The listing builds one solid part. Answer for the finished solid, in the listing's coordinates (mm). A direction names the side the tool comes from. Coordinates: 2 decimals unless noted, no trailing zeros. Loops run counter-clockwise (first coordinate to the right, second up) from the corner with the lowest first, then second, coordinate; pieces in that order, holes last. Notation, with made-up numbers: (-3, -8.5) - (45, -8.5) arc R12 cw to (45, 2.5) - close; hole circle Ø6 at (14.25, -8). An arc over 180 degrees is marked (long way). Put each result on its own line as item: value.
```python
from build123d import *

# Parameters (mm, degrees)
F0_W     = 12.7
F0_H     = 12.7
F1_DEPTH = 50.8
F2_DEPTH = 8.89
F3_F1_R  = 2.54
F3_F2_R  = 2.54


with BuildPart() as f1:
    # F0 (on Top) → F1 (new body)
    with BuildSketch(Plane.XY):
        Polygon((12.7, 12.7), (12.7, 0), (88.9, 0), (88.9, 12.7), (101.6, 12.7), (101.6, 88.9), (88.9, 88.9), (88.9, 101.6), (12.7, 101.6), (12.7, 88.9), (0, 88.9), (0, 12.7), align=None)
        with Locations((6.35, 95.25)):
            Rectangle(F0_W, F0_H)
        with Locations((95.25, 95.25)):
            Rectangle(F0_W, F0_H)
        with Locations((95.25, 6.35)):
            Rectangle(F0_W, F0_H)
        with Locations((6.35, 6.35)):
            Rectangle(F0_W, F0_H)
    extrude(amount=-F1_DEPTH)

    # F0 (on Top) → F2 (join)
    with BuildSketch(Plane.XY):
        Polygon((12.7, 12.7), (12.7, 0), (88.9, 0), (88.9, 12.7), (101.6, 12.7), (101.6, 88.9), (88.9, 88.9), (88.9, 101.6), (12.7, 101.6), (12.7, 88.9), (0, 88.9), (0, 12.7), align=None)
    extrude(amount=F2_DEPTH)

    # F3: fillet of radius 2.54 on 31 edges, made by hand

    # F3_f1
    f3_f1_edges = [f1.edges().sort_by_distance(p)[0] for p in [
        (88.9, 6.35, 0),
        (95.25, 12.7, 0),
        (88.9, 12.7, 4.445),
        (12.7, 12.7, 4.445),
        (6.35, 12.7, 0),
        (12.7, 6.35, 0),
        (12.7, 88.9, 4.445),
        (12.7, 95.25, 0),
        (6.35, 88.9, 0),
        (95.25, 88.9, 0),
        (88.9, 88.9, 4.445),
    ]]
    fillet(f3_f1_edges, radius=F3_F1_R)

    # F3_f2
    f3_f2_edges = [f1.edges().sort_by_distance(p)[0] for p in [
        (50.8, 101.6, 8.89),
        (0, 50.8, 8.89),
        (50.8, 0, 8.89),
        (96.52, 88.9, 8.89),
        (5.08, 88.9, 8.89),
        (5.08, 12.7, 8.89),
        (96.52, 12.7, 8.89),
        (101.6, 50.8, 8.89),
        (88.9, 5.08, 8.89),
        (12.7, 5.08, 8.89),
        (12.7, 96.52, 8.89),
        (88.9, 96.52, 8.89),
        (88.9, 101.6, 4.445),
        (101.6, 12.7, 5.715),
        (88.9, 0, 5.715),
        (12.7, 0, 5.715),
        (0, 12.7, 5.715),
        (0, 88.9, 5.715),
        (12.7, 101.6, 5.715),
        (101.6, 88.9, 5.715),
        (101.6, 89.6439487758, 0.7439487758),
        (11.9560512242, 101.6, 0.7439487758),
        (0, 89.6439487758, 0.7439487758),
        (0, 11.9560512242, 0.7439487758),
        (11.9560512242, 0, 0.7439487758),
        (89.6439487758, 0, 0.7439487758),
        (101.6, 11.9560512242, 0.7439487758),
        (89.6439487758, 89.6439487758, 8.89),
        (11.9560512242, 89.6439487758, 8.89),
        (11.9560512242, 11.9560512242, 8.89),
        (89.6439487758, 11.9560512242, 8.89),
    ]]
    fillet(f3_f2_edges, radius=F3_F2_R)


solid = f1.part
```
1) The part is cut by section B-B (y = 7.5). Give the vertices of the cut face in (x, z), and give its area (3 significant figures).
Found:
outline: (0, -50.8) - (101.6, -50.8) - (101.6, -2.54) arc R2.54 ccw to (99.06, 0) - (91.44, 0) arc R2.54 cw to (88.9, 2.54) - (88.9, 6.35) arc R2.54 ccw to (86.36, 8.89) - (15.24, 8.89) arc R2.54 ccw to (12.7, 6.35) - (12.7, 2.54) arc R2.54 cw to (10.16, 0) - (2.54, 0) arc R2.54 ccw to (0, -2.54) - close
area: 5,840 mm^2
2) For faces 1 (the face through (6.297, 89.664, 0.724)), 2 (the face through (88.136, 0.724, 4.472)), 3 (the face through (0.724, 5.151, -0.764)), determine the directions among +Z, -Z, +X, -X, +Y, -Y from which every point of the face is accessible in a straight line to the end or side of a thin tool.
Found:
face 1: +Z, -X, +Y
face 2: +Z, +X, -Y
face 3: +Z, -X, -Y
3) Each of these flat-tipped pins is pushed along its axis until it touches: pin 1 (1.1 mm diameter, centred on x = 96.5, z = 4, fed in from +Y); pin 2 (4 mm diameter, centred on y = 7, z = 3.5, fed in from +X); pin 3 (6 mm diameter, centred on x = 5.5, y = 5.5, fed in from +Z). Where does it stop, or does it pass through?
Found:
pin 1: stops at y = 88.9
pin 2: stops at x = 89.12
pin 3: stops at z = 0
4) The part is cut by section A-A (z = 5). Give the vertices of the cut face in (x, y).
Found:
outline: (0, 15.24) arc R2.54 ccw to (2.54, 12.7) - (10.16, 12.7) arc R2.54 cw to (12.7, 10.16) - (12.7, 2.54) arc R2.54 ccw to (15.24, 0) - (86.36, 0) arc R2.54 ccw to (88.9, 2.54) - (88.9, 10.16) arc R2.54 cw to (91.44, 12.7) - (99.06, 12.7) arc R2.54 ccw to (101.6, 15.24) - (101.6, 86.36) arc R2.54 ccw to (99.06, 88.9) - (91.44, 88.9) arc R2.54 cw to (88.9, 91.44) - (88.9, 99.06) arc R2.54 ccw to (86.36, 101.6) - (15.24, 101.6) arc R2.54 ccw to (12.7, 99.06) - (12.7, 91.44) arc R2.54 cw to (10.16, 88.9) - (2.54, 88.9) arc R2.54 ccw to (0, 86.36) - close
